from build123d import *

# Parameters (mm, degrees)
SKETCH_1_R          = 20
SKETCH_1_R_2        = 1.55
SKETCH_1_R_3        = 2.05
EXTRUDE_1_DEPTH     = 5
SKETCH_2_R          = 2.8
CUT_EXTRUDE_1_DEPTH = 3
SKETCH_3_R          = 3.5
CUT_EXTRUDE_2_DEPTH = 4
SKETCH_5_R          = 7.5
EXTRUDE_3_DEPTH     = 3.8
SKETCH_6_R          = 3
EXTRUDE_4_DEPTH     = 15
FILLET_1_R          = 2
SKETCH_7_R          = 3
SKETCH_7_R_2        = 2.7
CUT_EXTRUDE_3_DEPTH = 0.5


with BuildPart() as part:
    # 草图1 → 凸台-拉伸1 (new body)
    with BuildSketch(Plane.XY):
        Circle(SKETCH_1_R)
        with Locations((0, 15)):
            Circle(SKETCH_1_R_2, mode=Mode.SUBTRACT)
        with Locations((-11.313708499, 11.313708499)):
            Circle(SKETCH_1_R_3, mode=Mode.SUBTRACT)
        with Locations((11.313708499, 11.313708499)):
            Circle(SKETCH_1_R_3, mode=Mode.SUBTRACT)
        with Locations((15, 0)):
            Circle(SKETCH_1_R_2, mode=Mode.SUBTRACT)
        with Locations((11.313708499, -11.313708499)):
            Circle(SKETCH_1_R_3, mode=Mode.SUBTRACT)
        with Locations((0, -15)):
            Circle(SKETCH_1_R_2, mode=Mode.SUBTRACT)
        with Locations((-11.313708499, -11.313708499)):
            Circle(SKETCH_1_R_3, mode=Mode.SUBTRACT)
        with Locations((-15, 0)):
            Circle(SKETCH_1_R_2, mode=Mode.SUBTRACT)
    extrude(amount=EXTRUDE_1_DEPTH)

    # 草图2 → 切除-拉伸1 (cut)
    with BuildSketch(Plane.XY.offset(5)):
        with Locations((0, 15)):
            Circle(SKETCH_2_R)
        with Locations((15, 0)):
            Circle(SKETCH_2_R)
        with Locations((0, -15)):
            Circle(SKETCH_2_R)
        with Locations((-15, 0)):
            Circle(SKETCH_2_R)
    extrude(amount=-CUT_EXTRUDE_1_DEPTH, mode=Mode.SUBTRACT)

    # 草图3 → 切除-拉伸2 (cut)
    with BuildSketch(Plane.XY.offset(5)):
        with Locations((-11.313708499, 11.313708499)):
            Circle(SKETCH_3_R)
        with Locations((11.313708499, 11.313708499)):
            Circle(SKETCH_3_R)
        with Locations((11.313708499, -11.313708499)):
            Circle(SKETCH_3_R)
        with Locations((-11.313708499, -11.313708499)):
            Circle(SKETCH_3_R)
    extrude(amount=-CUT_EXTRUDE_2_DEPTH, mode=Mode.SUBTRACT)

    # 草图5 → 凸台-拉伸3 (add)
    with BuildSketch(Plane.XY.offset(5)):
        with Locations(Location((0, 0, 0), (0, 0, 180))):
            Circle(SKETCH_5_R)
    extrude(amount=EXTRUDE_3_DEPTH)

    # 草图6 → 凸台-拉伸4 (add)
    with BuildSketch(Plane.XY.offset(8.8)):
        Circle(SKETCH_6_R)
    extrude(amount=EXTRUDE_4_DEPTH)

    # 圆角1
    fillet_1_edges = [part.edges().sort_by_distance(p)[0] for p in [
        (7.5, 0, 5),
    ]]
    fillet(fillet_1_edges, radius=FILLET_1_R)

    # 草图7 → 切除-拉伸3 (cut)
    with BuildSketch(Plane.XY.offset(21.7)):
        Circle(SKETCH_7_R)
        Circle(SKETCH_7_R_2, mode=Mode.SUBTRACT)
    extrude(amount=CUT_EXTRUDE_3_DEPTH, mode=Mode.SUBTRACT)


solid = part.part
Source: CAD feature listing. Evaluate the final solid. Frame: model axes, mm. A direction names the side the tool comes from. Give positions to 0.01 mm unless a question says otherwise; leave off trailing zeros. Loops run counter-clockwise (first coordinate to the right, second up) from the corner with the lowest first, then second, coordinate; pieces in that order, holes last. Notation, with made-up numbers: (9.25, 61) -> (57.25, 61) arc R26 cw to (57.25, 89) -> close; hole circle Ø3 at (16.5, -3). An arc over 180 degrees is marked (long way). Use a Markdown table: item, result. Add a question column.
1) Section query B-B, the plane z = 15.5. Return the cut outline in (x, y), then the cut area to 3 significant figures.
2) Reachability of faces 4 (the face through (9.8, -9.93, 0.49)), 5 (the face through (-3, 0, 15)) from +Z, -Z, +X, -X, +Y, -Y: full face, straight path, thin tool, end or side. Return the list, or none.
3) First-contact query: pin 1 (3.5 mm diameter, centred on x = -11.31, y = -11.31, fed in from +Z); pin 2 (1.7 mm diameter, centred on x = 1, y = 15, fed in from +Z); pin 3 (10 mm diameter, centred on x = -1, z = 19, fed in from +Y); pin 4 (4 mm diameter, centred on x = 0.5, z = 4.5, fed in from -Y). Flat tips, straight axial feed; report the tip coordinate or a pass-through.
4) Pull-direction query (X, two-part tool) for faces 1 (the face through (-14.81, -11.16, 3.03)), 2 (the face through (-0.585, -2.636, 21.946)), 3 (the face through (9, -4, 5)); classes: +X half, -X half, draft (parallel to the pull), parting line (faces both ways), or undercut.
5) Section query C-C, the plane z = 7.75. Return the cut outline in (x, y), then the cut area to 3 significant figures.
6) Section query A-A, the plane x = 0. Count the separate pieces of the cut face and the enclosed holes in it, then the cut area to 3 significant figures.
7) Line query: line 1 along Y through (x, z) = (0, 4.25); line 2 along Z through (x, y) = (2, 6); line 3 along Y through (x, z) = (15, 3.85). Output: solid intervals per line, ascending. Write a range as [from, to].
Numbers:
| question | item | result |
|---|---|---|
| 1 | outline | circle Ø6 at (0, 0) |
| 1 | area | 28.3 mm2 |
| 2 | face 4 | +Z, -Z |
| 2 | face 5 | +Z |
| 3 | pin 1 | passes through |
| 3 | pin 2 | stops at z = 2 |
| 3 | pin 3 | stops at y = 3 |
| 3 | pin 4 | stops at y = -20 |
| 4 | face 1 | undercut |
| 4 | face 2 | parting line |
| 4 | face 3 | draft |
| 5 | outline | circle Ø15 at (0, 0) |
| 5 | area | 177 mm2 |
| 6 | separate pieces | 3 |
| 6 | enclosed holes | 0 |
| 6 | area | 302 mm2 |
| 7 | line 1 | y = [-20, -17.8], [-12.2, 12.2], [17.8, 20] |
| 7 | line 2 | z = [0, 8.8] |
| 7 | line 3 | y = [-13.23, -2.8], [2.8, 13.23] |
